Check sheet for the modelled part. Datum: model origin and axes. Units: mm. A direction names the side the tool comes from. Round coordinates to 2 decimals unless told otherwise and drop trailing zeros. Write each loop counter-clockwise with the first axis right and the second up, starting at its lowest first coordinate (ties: lowest second). Pieces come first, ordered by that corner, then holes. Notation, with made-up numbers: (-6, 26) -> (32, 26) arc R27 ccw to (32, 54) -> close; hole circle Ø9 at (56.5, 19). An arc over 180 degrees is marked (long way). Answer as a JSON object with one key per item and string values. Group by question number.
```python
from build123d import *

# Parameters (mm, degrees)
SKETCH1_W      = 27.95
SKETCH1_H      = 15.8
EXTRUDE1_DEPTH = 9.95
SKETCH2_R      = 1.5
EXTRUDE2_DEPTH = 10.95
FILLET1_R      = 2
SKETCH3_W      = 7
SKETCH3_H      = 1
EXTRUDE3_DEPTH = 11.5
SKETCH4_W      = 1
SKETCH4_H      = 7
EXTRUDE4_DEPTH = 3.5
SKETCH5_W      = 7
SKETCH5_H      = 1
EXTRUDE5_DEPTH = 9.5
SKETCH6_W      = 2.6
SKETCH6_H      = 4
EXTRUDE6_DEPTH = 3
SKETCH7_W      = 1
SKETCH7_H      = 3.836260464
EXTRUDE7_DEPTH = 3
SKETCH8_R      = 0.25
EXTRUDE8_DEPTH = 1


with BuildPart() as part:
    # Sketch1 → Extrude1 (new body)
    with BuildSketch(Plane.XY):
        Rectangle(SKETCH1_W, SKETCH1_H)
    extrude(amount=EXTRUDE1_DEPTH)

    # Sketch2 → Extrude2 (cut, through all)
    with BuildSketch(Plane.XY.offset(9.95)):
        with Locations((10.975, 4.9)):
            Circle(SKETCH2_R)
        with Locations((-10.975, -4.9)):
            Circle(SKETCH2_R)
    extrude(amount=-EXTRUDE2_DEPTH, mode=Mode.SUBTRACT)

    # Fillet1
    fillet1_edges = [part.edges().sort_by_distance(p)[0] for p in [
        (-13.975, 7.9, 4.975),
        (13.975, 7.9, 4.975),
        (13.975, -7.9, 4.975),
        (-13.975, -7.9, 4.975),
    ]]
    fillet(fillet1_edges, radius=FILLET1_R)

    # Sketch3 → Extrude3 (add)
    with BuildSketch(Plane.ZY.offset(13.975)):
        with Locations((4.975, -1.4)):
            Rectangle(SKETCH3_W, SKETCH3_H)
    extrude(amount=EXTRUDE3_DEPTH)

    # Sketch4 → Extrude4 (add)
    with BuildSketch(Plane(origin=(0, 7.9, 0), x_dir=(-1, 0, 0), z_dir=(0, 1, 0))):
        with Locations((1.175, 4.975)):
            Rectangle(SKETCH4_W, SKETCH4_H)
    extrude(amount=EXTRUDE4_DEPTH)

    # Sketch5 → Extrude5 (add)
    with BuildSketch(Plane.ZY.offset(1.675)):
        with Locations((4.975, 10.9)):
            Rectangle(SKETCH5_W, SKETCH5_H)
    extrude(amount=EXTRUDE5_DEPTH)

    # Sketch6 → Extrude6 (cut)
    with BuildSketch(Plane.XZ.offset(7.9)):
        with Locations((8.275, 4.975)):
            Rectangle(SKETCH6_W, SKETCH6_H)
    extrude(amount=-EXTRUDE6_DEPTH, mode=Mode.SUBTRACT)

    # Sketch7 → Extrude7 (cut)
    with BuildSketch(Plane.XZ.offset(7.9)):
        with Locations((-2.025, 5.414128699)):
            Rectangle(SKETCH7_W, SKETCH7_H)
    extrude(amount=-EXTRUDE7_DEPTH, mode=Mode.SUBTRACT)

    # Sketch8 → Extrude8 (cut)
    with BuildSketch(Plane(origin=(0, 0, 7.332258931), x_dir=(-1, 0, 0), z_dir=(0, 0, -1))):
        with Locations((2.025, -5.4)):
            Circle(SKETCH8_R)
    extrude(amount=-EXTRUDE8_DEPTH, mode=Mode.SUBTRACT)


solid = part.part
```
(1) Go/stop test with flat-tipped pins: pin 1 Ø0.8 at (x, y) = (-17.5, -1.5) entering from -Z (3 decimals); pin 2 Ø3 at (y, z) = (9, 6) entering from +X (3 decimals); pin 3 Ø4 at (x, y) = (-8.5, 9.5) entering from -Z; pin 4 Ø0.8 at (x, z) = (8.5, 5.5) entering from -Y. Record where each tip stops, or that it passes through.
(2) Section check C-C on x = 1. Record the cut outline in (y, z), then the cut area to 3 significant figures.
(3) Section check A-A on y = 4.9. Record the cut outline in (x, z) (3 decimals), then the cut area to 3 significant figures.
(4) Section check D-D on y = 2.75. Record the cut outline in (x, z) (3 decimals).
(5) Access from +Z, -Z, +X, -X, +Y, -Y to the whole of each face (thin tool, end or side, straight path). Record for faces 4 (the flat face through (-19.6, -1.4, 1.475)), 5 (the flat face through (-1.525, -6, 5)), 6 (the flat face through (-0.675, 10, 5)), 7 (the flat face through (-20, -1.9, 5)).
(6) Scan lines: line 1 along X through (y, z) = (-5.5, 6.75) (3 decimals); line 2 along Y through (x, z) = (-3.5, 6.75); line 3 along X through (y, z) = (2.5, 7) (3 decimals). Record each from-to range of solid material in increasing order.
(7) Release check for a two-part mould opening along Z. For faces 1 (the flat face through (0, 0, 0)), 2 (the flat face through (-6, 11.4, 5)), 3 (the flat face through (8, -4.9, 5)) record: pulls with the +Z half, pulls with the -Z half, needs draft (parallel to the pull), parting line crosses it, or undercut.
(8) Section check B-B on z = 4.25. Record the cut outline in (x, y) (3 decimals), then the cut area to 3 significant figures.
Data:
{
 "1": {"pin 1": "stops at z = 1.475", "pin 2": "stops at x = 13.175", "pin 3": "stops at z = 0", "pin 4": "stops at y = -4.9"},
 "2": {"outline": "(-7.9, 0) -> (7.9, 0) -> (7.9, 9.95) -> (-7.9, 9.95) -> close", "area": "157 mm²"},
 "3": {"outline": "(-13.975, 0) -> (9.475, 0) -> (9.475, 9.95) -> (-13.975, 9.95) -> close; (12.475, 0) -> (13.975, 0) -> (13.975, 9.95) -> (12.475, 9.95) -> close", "area": "248 mm²"},
 "4": {"outline": "(-13.975, 0) -> (13.975, 0) -> (13.975, 9.95) -> (-13.975, 9.95) -> close"},
 "5": {"face 4": "-Z, -X, +Y, -Y", "face 5": "-Y", "face 6": "+Z, -Z, +X, +Y", "face 7": "+Z, -Z, -X, -Y"},
 "6": {"line 1": "x = -13.975 to -12.35, -9.6 to -2.525, -1.525 to 6.975, 9.575 to 13.975", "line 2": "y = -7.9 to 7.9, 10.4 to 11.4", "line 3": "x = -13.975 to 13.975"},
 "7": {"face 1": "pulls with the -Z half", "face 2": "needs draft", "face 3": "undercut"},
 "8": {"outline": "(-25.475, -1.9) -> (-13.975, -1.9) -> (-13.975, -5.9) arc R2 ccw to (-11.975, -7.9) -> (-2.525, -7.9) -> (-2.525, -4.9) -> (-1.525, -4.9) -> (-1.525, -7.9) -> (6.975, -7.9) -> (6.975, -4.9) -> (9.575, -4.9) -> (9.575, -7.9) -> (11.975, -7.9) arc R2 ccw to (13.975, -5.9) -> (13.975, 5.9) arc R2 ccw to (11.975, 7.9) -> (-0.675, 7.9) -> (-0.675, 11.4) -> (-11.175, 11.4) -> (-11.175, 10.4) -> (-1.675, 10.4) -> (-1.675, 7.9) -> (-11.975, 7.9) arc R2 ccw to (-13.975, 5.9) -> (-13.975, -0.9) -> (-25.475, -0.9) -> close; hole circle Ø3 at (-10.975, -4.9); hole circle Ø3 at (10.975, 4.9)", "area": "438 mm²"}
}
